Check sheet for the modelled part. Datum: model origin and axes. Units: mm. A direction names the side the tool comes from. Coordinates: 2 decimals unless noted, no trailing zeros. Loops run counter-clockwise (first coordinate to the right, second up) from the corner with the lowest first, then second, coordinate; pieces in that order, holes last.
from build123d import *

# Parameters (mm, degrees)
SKETCH1_R           = 6.4
BOSS_EXTRUDE1_DEPTH = 5
SKETCH7_R           = 1.5
CUT_EXTRUDE4_DEPTH  = 10
BOSS_EXTRUDE2_DEPTH = 10
BOSS_EXTRUDE3_DEPTH = 4
FILLET1_R           = 2
FILLET2_R           = 2
SKETCH12_R          = 1.5
CUT_EXTRUDE5_DEPTH  = 13
SKETCH13_W          = 8.5
SKETCH13_H          = 8
CUT_EXTRUDE6_DEPTH  = 13
SKETCH13_3_R        = 3
SKETCH13_3_W        = 13
SKETCH13_3_H        = 8
CUT_EXTRUDE7_DEPTH  = 1.75
SKETCH15_R          = 1
CUT_EXTRUDE9_DEPTH  = 10


with BuildPart() as part:
    # Sketch1 → Boss-Extrude1 (new body)
    with BuildSketch(Plane(origin=(0, 0, 0), x_dir=(1, 0, 0), z_dir=(0, 1, 0))):
        with BuildLine():
            ThreePointArc((54.302519507, -4.751051874), (55.339723673, -0.00587799), (54.307413406, 4.740362963))
            Line((54.307413406, 4.740362963), (37.5, 41.5))
            Line((37.5, 41.5), (-67.5, 41.5))
            Line((-67.5, 41.5), (-67.5, -41.4))
            Line((-67.5, -41.4), (37.5, -41.4))
            Line((37.5, -41.4), (54.302519507, -4.751051874))
        make_face()
        with Locations(Location((43.939725188, 0, 0), (0, 0, 270))):
            Circle(SKETCH1_R, mode=Mode.SUBTRACT)
    extrude(amount=BOSS_EXTRUDE1_DEPTH)

    # Sketch7 → Cut-Extrude4 (cut)
    with BuildSketch(Plane.XZ):
        with Locations(Location((-34.6, 36.9, 0), (0, 0, 270))):
            Circle(SKETCH7_R)
        with Locations(Location((-63.5, 36.9, 0), (0, 0, 270))):
            Circle(SKETCH7_R)
        with Locations(Location((-63.5, -37, 0), (0, 0, 270))):
            Circle(SKETCH7_R)
        with Locations(Location((-34.6, -37, 0), (0, 0, 270))):
            Circle(SKETCH7_R)
    extrude(amount=-CUT_EXTRUDE4_DEPTH, mode=Mode.SUBTRACT)

    # Sketch9 → Boss-Extrude2 (add)
    with BuildSketch(Plane.XZ):
        Polygon((-35.7, 26.505), (-62.5, 26.505), (-62.5, 23.505), (-38.7, 23.505), (-38.7, -20.995), (-62.5, -20.995), (-62.5, -23.995), (-35.7, -23.995), align=None)
    extrude(amount=BOSS_EXTRUDE2_DEPTH)

    # Sketch9<3> → Boss-Extrude3 (add)
    with BuildSketch(Plane.XZ):
        Polygon((-62.5, 26.505), (-64.5, 26.505), (-64.5, 21.505), (-62.5, 23.505), align=None)
        Polygon((-64.5, -18.995), (-64.5, -23.995), (-62.5, -23.995), (-62.5, -20.995), align=None)
    extrude(amount=BOSS_EXTRUDE3_DEPTH)

    # Fillet1
    fillet1_edges = [part.edges().sort_by_distance(p)[0] for p in [
        (-62.5, -4, 25.005),
        (-62.5, -4, -22.495),
    ]]
    fillet(fillet1_edges, radius=FILLET1_R - 0.0001)  # a hair under: the kernel refuses the full size

    # Fillet2
    fillet2_edges = [part.edges().sort_by_distance(p)[0] for p in [
        (-35.7, -5, 26.505),
        (-35.7, -5, -23.995),
    ]]
    fillet(fillet2_edges, radius=FILLET2_R)

    # Sketch12 → Cut-Extrude5 (cut)
    with BuildSketch(Plane.XZ):
        with Locations(Location((32.4, 11.85, 0), (0, 0, 270))):
            Circle(SKETCH12_R)
        with Locations(Location((32.4, -11.95, 0), (0, 0, 270))):
            Circle(SKETCH12_R)
        with Locations(Location((3.115937957, -17.546796564, 0), (0, 0, 270))):
            Circle(SKETCH12_R)
        with Locations(Location((-13.713203436, -34.375937957, 0), (0, 0, 270))):
            Circle(SKETCH12_R)
        with Locations(Location((3.115937957, 17.446796564, 0), (0, 0, 270))):
            Circle(SKETCH12_R)
        with Locations(Location((-13.713203436, 34.275937957, 0), (0, 0, 270))):
            Circle(SKETCH12_R)
    extrude(amount=-CUT_EXTRUDE5_DEPTH, mode=Mode.SUBTRACT)

    # Sketch13 → Cut-Extrude6 (cut)
    with BuildSketch(Plane.XZ):
        with Locations((3.75, 0)):
            Rectangle(SKETCH13_W, SKETCH13_H)
    extrude(amount=-CUT_EXTRUDE6_DEPTH, mode=Mode.SUBTRACT)

    # Sketch13<3> → Cut-Extrude7 (cut)
    with BuildSketch(Plane.XZ):
        with Locations((-3.85, 0)):
            Circle(SKETCH13_3_R)
        with Locations((1.5, 0)):
            Rectangle(SKETCH13_3_W, SKETCH13_3_H)
    extrude(amount=-CUT_EXTRUDE7_DEPTH, mode=Mode.SUBTRACT)

    # Sketch15 → Cut-Extrude9 (cut)
    with BuildSketch(Plane.XZ.offset(-1.75)):
        with Locations(Location((-2.85, 0, 0), (0, 0, 270))):
            Circle(SKETCH15_R)
    extrude(amount=-CUT_EXTRUDE9_DEPTH, mode=Mode.SUBTRACT)


solid = part.part
(1) Scan lines: line 1 along X through (y, z) = (1.5, 36.9); line 2 along Y through (x, z) = (-60.5, 30); line 3 along X through (y, z) = (-5, 16). Record each from-to range of solid material in increasing order.
(2) Draft check along Z on faces 1 (the face through (-35.7, -5, 1)), 2 (the face through (30.936, 2.465, -11.625)), 3 (the face through (-51, -5, -23.995)), 4 (the face through (-14.29, 2.46, -35.76)). Enter one of: pulls with the +Z half, pulls with the -Z half, needs draft (parallel to the pull), parting line crosses it, or undercut.
(3) Section check D-D, the plane z = 11.85. Enter the section's corners in (x, y), plus the area to 3 significant figures.
(4) Section check A-A, the plane x = 32.4. Enter the section's corners in (y, z), plus the area to 4 significant figures.
(5) Gauge pin test, flat ends, axial feed: P1, Ø2.5, axis at x = 32.4, z = 11.85, coming from the +Y side; P2, Ø3, axis at x = -53, y = -6.5, coming from the +Z side (3 decimals); P3, Ø3, axis at y = -2, z = -22.5, coming from the -X side; P4, Ø1, axis at x = -39.5, y = -8, coming from the -Z side (3 decimals). Record the tip position at first contact, or that the pin passes through.
(6) Section check B-B, the plane y = -1.75. Enter the section's corners in (x, z) (3 decimals).
(7) Set-up check for faces 5 (the face through (-51, -5, 26.505)), 6 (the face through (-62.5, -8, 25)), 7 (the face through (-4, 1.75, -1)): record each of +Z, -Z, +X, -X, +Y, -Y from which the full face is reachable in a straight line by a thin tool's end or side.
(8) Section check C-C, the plane x = -49.5. Enter the section's corners in (y, z) (3 decimals), plus the area to 4 significant figures.
Determined:
1. line 1: x = -67.5 to -65, -62 to -36.1, -33.1 to 39.56
1. line 2: y = 0 to 5
1. line 3: x = -38.7 to -35.7
2. face 1: needs draft
2. face 2: undercut
2. face 3: pulls with the -Z half
2. face 4: undercut
3. outline: (-67.5, 0) - (-38.7, 0) - (-38.7, -10) - (-35.7, -10) - (-35.7, 0) - (30.9, 0) - (30.9, 5) - (-67.5, 5) - close; (33.9, 0) - (51.05, 0) - (51.05, 5) - (33.9, 5) - close
3. area: 608 mm2
4. outline: (0, -41.5) - (5, -41.5) - (5, -13.45) - (0, -13.45) - close; (0, -10.45) - (5, -10.45) - (5, 10.35) - (0, 10.35) - close; (0, 13.35) - (5, 13.35) - (5, 41.4) - (0, 41.4) - close
4. area: 384.5 mm2
5. P1: passes through
5. P2: stops at z = 26.505
5. P3: stops at x = -64.5
5. P4: stops at z = -23.995
6. outline: (-64.5, -23.995) - (-37.7, -23.995) arc R2 ccw to (-35.7, -21.995) - (-35.7, 24.505) arc R2 ccw to (-37.7, 26.505) - (-64.5, 26.505) - (-64.5, 21.505) - (-62.5, 23.505) - (-38.7, 23.505) - (-38.7, -20.995) - (-62.5, -20.995) - (-64.5, -18.995) - close
7. face 5: +Z, +X, -X, -Y
7. face 6: +Z, -Z, -X, -Y
7. face 7: -Y
8. outline: (-10, -23.995) - (0, -23.995) - (0, -41.5) - (5, -41.5) - (5, 41.4) - (0, 41.4) - (0, 26.505) - (-10, 26.505) - (-10, 23.505) - (0, 23.505) - (0, -20.995) - (-10, -20.995) - close
8. area: 474.5 mm2
